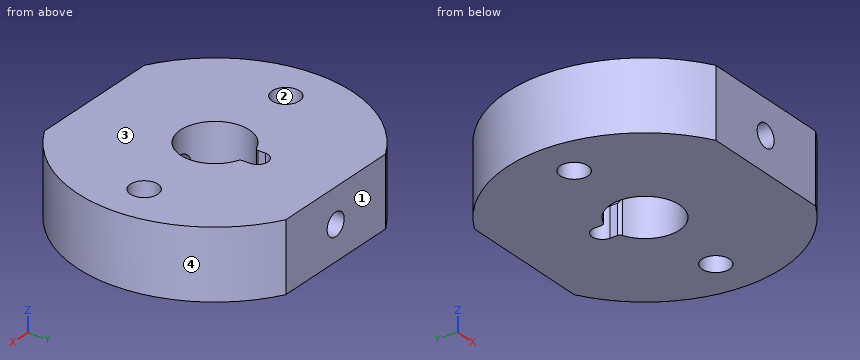
```python
from build123d import *

# Parameters (mm, degrees)
SKETCH_1_R               = 20
SKETCH_1_R_2             = 5
SKETCH_1_R_3             = 1.9999999999999996
SKETCH_1_R_4             = 2.0000000000000013
EXTRUDE_1_DEPTH          = 10
CUT_EXTRUDE_1_DEPTH      = 31
CUT_EXTRUDE_1_DEPTH_BACK = 31
SKETCH_2_R               = 1.6500000000000001
CUT_EXTRUDE_2_DEPTH      = 31.00000018509541
CUT_EXTRUDE_3_DEPTH      = 31.00000018509541
FILLET_1_R               = 0.5


with BuildPart() as part:
    # ｽｹｯﾁ1 → ﾎﾞｽ - 押し出し1 (new body)
    with BuildSketch(Plane.XY):
        Circle(SKETCH_1_R)
        Circle(SKETCH_1_R_2, mode=Mode.SUBTRACT)
        with Locations((-13.75, 0)):
            Circle(SKETCH_1_R_3, mode=Mode.SUBTRACT)
        with Locations((13.75, 0)):
            Circle(SKETCH_1_R_4, mode=Mode.SUBTRACT)
    extrude(amount=EXTRUDE_1_DEPTH)

    # ｽｹｯﾁ2 → ｶｯﾄ - 押し出し1 (cut, two sides: drawn at the far end of the back side and taken through both)
    with BuildSketch(Plane(origin=(0, 0, 0), x_dir=(1, 0, 0), z_dir=(0, 1, 0)).offset(-CUT_EXTRUDE_1_DEPTH_BACK)):
        with Locations(Location((0, -5, 0), (0, 0, 270))):
            Circle(SKETCH_2_R)
    extrude(amount=CUT_EXTRUDE_1_DEPTH + CUT_EXTRUDE_1_DEPTH_BACK, mode=Mode.SUBTRACT)

    # ｽｹｯﾁ3 → ｶｯﾄ - 押し出し2 (cut, through all)
    with BuildSketch(Plane.XY.offset(10)):
        with BuildLine():
            ThreePointArc((-0.8423325125714249, 4.928536896307575), (-0.42267926283542223, 4.982102190919903), (-8.296e-14, 5))
            Line((0, 5), (0, 6.169696007084729))
            Line((0, 6.169696007084729), (-1.5, 6.169696007084729))
            ThreePointArc((-1.5000000000000002, 6.169696007084729), (-1.3254242280977697, 5.4673779768652055), (-0.8423325125714237, 4.928536896307585))
        make_face()
        with BuildLine():
            Line((0, 6.169696007084729), (0, 5))
            ThreePointArc((-8.296e-14, 5), (0.42267926283533985, 4.982102190919911), (0.8423325125714245, 4.928536896307575))
            ThreePointArc((0.8423325125714223, 4.928536896307583), (1.325424228097769, 5.467377976865205), (1.5000000000000002, 6.169696007084729))
            Line((1.5, 6.169696007084729), (0, 6.169696007084729))
        make_face()
        with BuildLine():
            Line((-1.5, 6.169696007084729), (0, 6.169696007084729))
            Line((0, 6.169696007084729), (0, 7.669696007084729))
            ThreePointArc((1.974e-14, 7.669696007084729), (-1.0606601717798143, 7.230356178864558), (-1.5000000000000002, 6.169696007084729))
        make_face()
        with BuildLine():
            Line((0, 7.669696007084729), (0, 6.169696007084729))
            Line((0, 6.169696007084729), (1.5, 6.169696007084729))
            ThreePointArc((1.5000000000000002, 6.169696007084729), (1.0606601717798283, 7.230356178864544), (1.941e-14, 7.669696007084729))
        make_face()
        with BuildLine():
            Line((-1.5, 6.169696007084729), (0, 6.169696007084729))
            Line((0, 6.169696007084729), (0, 7.669696007084729))
            ThreePointArc((1.974e-14, 7.669696007084729), (-1.0606601717798143, 7.230356178864558), (-1.5000000000000002, 6.169696007084729))
        make_face()
        with BuildLine():
            Line((0, 7.669696007084729), (0, 6.169696007084729))
            Line((0, 6.169696007084729), (1.5, 6.169696007084729))
            ThreePointArc((1.5000000000000002, 6.169696007084729), (1.0606601717798283, 7.230356178864544), (1.941e-14, 7.669696007084729))
        make_face()
        with BuildLine():
            ThreePointArc((0.8423325125714245, 4.928536896307575), (1.173856041806049, 4.860253284872655), (1.4999999999999996, 4.769696007084728))
            Line((1.5, 4.769696007084729), (1.5, 6.169696007084729))
            ThreePointArc((1.5000000000000002, 6.169696007084729), (1.325424228097769, 5.467377976865205), (0.8423325125714223, 4.928536896307583))
        make_face()
        with BuildLine():
            ThreePointArc((-0.8423325125714249, 4.928536896307575), (-0.42267926283542223, 4.982102190919903), (-8.296e-14, 5))
            Line((0, 5), (0, 6.169696007084729))
            Line((0, 6.169696007084729), (-1.5, 6.169696007084729))
            ThreePointArc((-1.5000000000000002, 6.169696007084729), (-1.3254242280977697, 5.4673779768652055), (-0.8423325125714237, 4.928536896307585))
        make_face()
        with BuildLine():
            Line((0, 6.169696007084729), (0, 5))
            ThreePointArc((-8.296e-14, 5), (0.42267926283533985, 4.982102190919911), (0.8423325125714245, 4.928536896307575))
            ThreePointArc((0.8423325125714223, 4.928536896307583), (1.325424228097769, 5.467377976865205), (1.5000000000000002, 6.169696007084729))
            Line((1.5, 6.169696007084729), (0, 6.169696007084729))
        make_face()
        with BuildLine():
            Line((-1.5, 6.169696007084729), (-1.5, 4.769696007084729))
            ThreePointArc((-1.5, 4.769696007084728), (-1.1738560418060509, 4.8602532848726545), (-0.8423325125714249, 4.928536896307575))
            ThreePointArc((-0.8423325125714237, 4.928536896307585), (-1.3254242280977697, 5.4673779768652055), (-1.5000000000000002, 6.169696007084729))
        make_face()
    extrude(amount=-CUT_EXTRUDE_2_DEPTH, mode=Mode.SUBTRACT)

    # ｽｹｯﾁ4 → ｶｯﾄ - 押し出し3 (cut, through all)
    with BuildSketch(Plane.XY.offset(10)):
        with BuildLine():
            ThreePointArc((9.68245836551855, 17.499999999999996), (1.22e-15, 20), (-9.682458365518547, 17.499999999999996))
            Line((-9.682458365518546, 17.499999999999996), (9.68245836551855, 17.499999999999996))
        make_face()
        with BuildLine():
            Line((9.68245836551855, -17.499999999999996), (-9.682458365518546, -17.499999999999996))
            ThreePointArc((-9.682458365518551, -17.499999999999996), (-3.67e-15, -20), (9.682458365518546, -17.499999999999996))
        make_face()
    extrude(amount=-CUT_EXTRUDE_3_DEPTH, mode=Mode.SUBTRACT)

    # ﾌｨﾚｯﾄ1
    fillet_1_edges = [part.edges().sort_by_distance(p)[0] for p in [
        (1.4999999999999998, 4.769696007084728, 7.843693197647017),
        (-1.5, 4.769696007084729, 7.843693197355676),
    ]]
    fillet(fillet_1_edges, radius=FILLET_1_R)


solid = part.part
```
Build history of the part. All positions in model axes, mm. Face numbers are marked on the shaded views. Round coordinates to 2 decimals unless told otherwise and drop trailing zeros. Write each loop counter-clockwise with the first axis right and the second up, starting at its lowest first coordinate (ties: lowest second). Pieces come first, ordered by that corner, then holes.
1) Drill centre lines: probe 1 along Z at (x, y) = (0, 14.5); probe 2 along Y at (x, z) = (0, 2.5); probe 3 along Y at (x, z) = (-13.5, 1.5). Where is each one in solid material? Low to high.
2) Band-saw the part on A-A, the plane z = 5. List the corners of the cut face in (x, y).
3) Pin check, flat tips, straight feed: pin 1 (2.5 mm diameter, centred on x = 0, z = 5, fed in from +Y); pin 2 (1 mm diameter, centred on y = -6, z = 2, fed in from +X); pin 3 (1.2 mm diameter, centred on y = 5.5, z = 2, fed in from +X); pin 4 (0.8 mm diameter, centred on y = 5.5, z = 7, fed in from -X). Stop position of each tip, or through.
4) Band-saw the part on D-D, the plane y = 1.5. List the corners of the cut face in (x, z).
5) Band-saw the part on B-B, the plane x = 0. List the corners of the cut face in (y, z), and give its area (3 significant figures).
6) Mould opens along Y. For the marked faces 1, 2, 3 and 4 say: +Y half, -Y half, draft (parallel to the pull), parting line (faces both ways), or undercut.
7) Band-saw the part on C-C, the plane x = -13.75. List the corners of the cut face in (y, z), and give its area (3 significant figures).
Ans:
1. probe 1: z = 0 to 3.35, 6.65 to 10
1. probe 2: y = -17.5 to -5, 7.67 to 17.5
1. probe 3: y = -14.76 to -1.98, 1.98 to 14.76
2. outline: (-9.68, -17.5) - (-1.65, -17.5) - (-1.65, -4.72) arc R5 cw to (-1.82, 4.66) arc R0.5 ccw to (-1.65, 4.77) - (-1.65, 17.5) - (-9.68, 17.5) arc R20 ccw to start; (1.65, -17.5) - (9.68, -17.5) arc R20 ccw to (9.68, 17.5) - (1.65, 17.5) - (1.65, 4.77) arc R0.5 ccw to (1.82, 4.66) arc R5 cw to (1.65, -4.72) - close; hole circle Ø4 at (-13.75, 0); hole circle Ø4 at (13.75, 0)
3. pin 1: passes through
3. pin 2: stops at x = 19.23
3. pin 3: stops at x = 19.39
3. pin 4: stops at x = -19.34
4. outline: (-19.94, 0) - (-15.07, 0) - (-15.07, 10) - (-19.94, 10) - close; (-12.43, 0) - (-4.77, 0) - (-4.77, 10) - (-12.43, 10) - close; (4.77, 0) - (12.43, 0) - (12.43, 10) - (4.77, 10) - close; (15.07, 0) - (19.94, 0) - (19.94, 10) - (15.07, 10) - close
5. outline: (-17.5, 0) - (-5, 0) - (-5, 3.35) - (-17.5, 3.35) - close; (-17.5, 6.65) - (-5, 6.65) - (-5, 10) - (-17.5, 10) - close; (7.67, 0) - (17.5, 0) - (17.5, 3.35) - (7.67, 3.35) - close; (7.67, 6.65) - (17.5, 6.65) - (17.5, 10) - (7.67, 10) - close
5. area: 150 mm2
6. face 1: +Y half
6. face 2: undercut
6. face 3: draft
6. face 4: parting line
7. outline: (-14.52, 0) - (-2, 0) - (-2, 10) - (-14.52, 10) - close; (2, 0) - (14.52, 0) - (14.52, 10) - (2, 10) - close
7. area: 250 mm2
